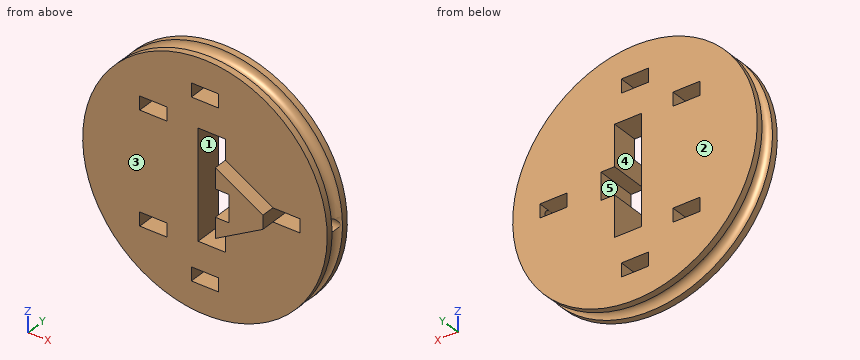
```python
from build123d import *

# Parameters (mm, degrees)
CROQUIS2_W              = 10
CROQUIS2_H              = 5
CORTAR_EXTRUIR1_DEPTH   = 10
CROQUIS3_R              = 2.5
CORTAR_EXTRUIR2_DEPTH   = 50
SALIENTE_EXTRUIR1_DEPTH = 15
CROQUIS5_W              = 10
CROQUIS5_H              = 5
CORTAR_EXTRUIR3_DEPTH   = 10


with BuildPart() as part:
    # Croquis1 → Revolución1 (revolve)
    with BuildSketch(Plane(origin=(0, 0, 0), x_dir=(0, 0, -1), z_dir=(1, 0, 0))):
        with BuildLine():
            Line((-45, 2.6), (-45, 5))
            Line((-45, 5), (0, 5))
            Line((0, 5), (0, -5))
            Line((0, -5), (-45, -5))
            Line((-45, -5), (-45, -2.6))
            ThreePointArc((-45, -2.6), (-42.4, 0), (-45, 2.6))
        make_face()
    revolve(axis=Axis((0, 59.07084426, 0), (0, -1, 0)))

    # Croquis2 → Cortar-Extruir1 (cut)
    with BuildSketch(Plane(origin=(0, 5, 0), x_dir=(1, 0, 0), z_dir=(0, 1, 0))):
        Polygon((7.5, 5), (7.5, 20), (-2.5, 20), (-2.5, -20), (7.5, -20), (7.5, -5), (12.5, -5), (12.5, 5), align=None)
        with Locations((0, 32.5)):
            Rectangle(CROQUIS2_W, CROQUIS2_H)
        with Locations((0, -32.5)):
            Rectangle(CROQUIS2_W, CROQUIS2_H)
        with Locations((30, 0)):
            Rectangle(CROQUIS2_W, CROQUIS2_H)
    extrude(amount=-CORTAR_EXTRUIR1_DEPTH, mode=Mode.SUBTRACT)

    # Croquis3 → Cortar-Extruir2 (cut)
    with BuildSketch(Plane.ZY.offset(-12.5)):
        Circle(CROQUIS3_R)
    extrude(amount=-CORTAR_EXTRUIR2_DEPTH, mode=Mode.SUBTRACT)

    # Croquis4 → Saliente-Extruir1 (add)
    with BuildSketch(Plane(origin=(0, 5, 0), x_dir=(1, 0, 0), z_dir=(0, 1, 0))):
        Polygon((7.5, 12.5), (25, 2.5), (25, -2.5), (7.5, -12.5), (7.5, -5), (12.5, -5), (12.5, 5), (7.5, 5), align=None)
    extrude(amount=-SALIENTE_EXTRUIR1_DEPTH)

    # Croquis5 → Cortar-Extruir3 (cut)
    with BuildSketch(Plane(origin=(0, 5, 0), x_dir=(1, 0, 0), z_dir=(0, 1, 0))):
        with Locations((-19, -20.5)):
            Rectangle(CROQUIS5_W, CROQUIS5_H)
        with Locations((-19, 20.5)):
            Rectangle(CROQUIS5_W, CROQUIS5_H)
    extrude(amount=-CORTAR_EXTRUIR3_DEPTH, mode=Mode.SUBTRACT)


solid = part.part
```
Check sheet for the modelled part. Datum: model origin and axes. Units: mm. Face numbers are marked on the shaded views. A direction names the side the tool comes from. Give positions to 0.01 mm unless a question says otherwise; leave off trailing zeros. Order: outer loops, then holes, each group sorted by start corner. A loop starts at its lowest first (then second) coordinate and runs counter-clockwise, first axis right, second up. Notation, with made-up numbers: (-36, 23.25) -> (-3, 23.25) arc R7 cw to (-3, 28.25) -> close; hole circle Ø8 at (79, 52.25). An arc over 180 degrees is marked (long way). Use CSV: the item, a comma, the result in double quotes. Start each with the question number.
1) Sectioned sample at B-B, the plane z = 0. Record the boundary of the cut face in (x, y), plus the area to 3 significant figures.
2) Sectioned sample at A-A, the plane x = 0. Record the boundary of the cut face in (y, z).
3) Go/stop test with flat-tipped pins: P1, Ø1, axis at x = -24.5, z = 25.5, coming from the -Y side; P2, Ø3, axis at x = 1, y = 0.5, coming from the -Z side; P3, Ø5, axis at y = -0.5, z = -7.5, coming from the +X side; P4, Ø5, axis at x = 0, y = 0.5, coming from the +Z side. Record where each tip stops, or that it passes through.
4) Sectioned sample at D-D, the plane x = -20. Give the number of separate pieces and of enclosed holes in the cut face, plus the area to 3 significant figures.
5) Sectioned sample at C-C, the plane y = -6.5. Record the boundary of the cut face in (x, z).
6) Mould release check, pull along Z, two halves, no side actions. Record for the marked faces 3, 4 and 5: released by +Z, released by -Z, zero draft, split by the parting line, or undercut.
7) Set-up check for the marked faces 1 and 2: record each of +Z, -Z, +X, -X, +Y, -Y from which the full face is reachable in a straight line by a thin tool's end or side.
8) Material ranges on line 1 (Y direction, x = 39.5, z = 0); line 2 (Z direction, x = -22, y = 2); line 3 (Z direction, x = -23, y = 2), recorded low to high. Write a range as from..to.
Recorded:
1,outline,"(-45, -5) -> (-2.5, -5) -> (-2.5, 5) -> (-45, 5) -> (-45, 2.6) arc R2.6 cw to (-45, -2.6) -> close; (12.5, -10) -> (25, -10) -> (25, 5) -> (12.5, 5) -> close; (35, -5) -> (45, -5) -> (45, -2.6) arc R2.6 cw to (44.29, -2.5) -> (35, -2.5) -> close; (35, 2.5) -> (44.29, 2.5) arc R2.6 cw to (45, 2.6) -> (45, 5) -> (35, 5) -> close"
1,area,"652 mm2"
2,outline,"(-5, -45) -> (-2.6, -45) arc R2.6 cw to (2.6, -45) -> (5, -45) -> (5, -35) -> (-5, -35) -> close; (-5, -30) -> (5, -30) -> (5, -20) -> (-5, -20) -> close; (-5, 20) -> (5, 20) -> (5, 30) -> (-5, 30) -> close; (-5, 35) -> (5, 35) -> (5, 45) -> (2.6, 45) arc R2.6 cw to (-2.6, 45) -> (-5, 45) -> close"
3,P1,"y = -5"
3,P2,"z = -43.33"
3,P3,"x = 44.58"
3,P4,"z = 45"
4,separate pieces,"3"
4,enclosed holes,"0"
4,area,"682 mm2"
5,outline,"(7.5, -12.5) -> (25, -2.5) -> (25, 2.5) -> (7.5, 12.5) -> (7.5, 5) -> (12.5, 5) -> (12.5, -5) -> (7.5, -5) -> close"
6,face 3,"zero draft"
6,face 4,"undercut"
6,face 5,"undercut"
7,face 1,"+Y, -Y"
7,face 2,"+Z, -Z, +X, -X, +Y"
8,line 1,"-5..-2.5, 2.5..5"
8,line 2,"-37.34..-23, -18..18, 23..37.34"
8,line 3,"-36.73..-23, -18..18, 23..36.73"
